Source: CAD feature listing. Evaluate the final solid. Frame: model axes, mm. Face numbers are marked on the shaded views. A direction names the side the tool comes from. Round coordinates to 2 decimals unless told otherwise and drop trailing zeros. Write each loop counter-clockwise with the first axis right and the second up, starting at its lowest first coordinate (ties: lowest second). Pieces come first, ordered by that corner, then holes. Notation, with made-up numbers: (-1, 8) -> (38, 8) arc R21 ccw to (38, 16) -> close; hole circle Ø2 at (40.25, 54.5). An arc over 180 degrees is marked (long way). Put each result on its own line as item: value.
Autodesk Inventor part; units mm, degrees
ref_plane "YZ Plane" through (0, 0, 0) normal (1, 0, 0) x (0, 1, 0)
ref_plane "XZ Plane" through (0, 0, 0) normal (0, 1, 0) x (-1, 0, 0)
ref_plane "XY Plane" through (0, 0, 0) normal (0, 0, 1) x (1, 0, 0)
sketch "Sketch1" plane through (0, 0, 0) normal (0, 1, 0) x (-1, 0, 0)
  line L0 (0, 0) -> (27, 0) construction
  line L1 (27, 0) -> (27, -25) construction
  line L2 (27, -25) -> (0, -25) construction
  line L3 (0, -25) -> (0, 0) construction
  line L4 (31, 2) -> (-4, 2)
  line L5 (-4, -27) -> (31, -27)
  line L6 (29, -22) -> (29, -3)
  line L7 (28, -4) -> (23.5, -4)
  line L8 (23.5, -4) -> (23.5, -21)
  line L9 (23.5, -21) -> (28, -21)
  line L10 (28, -21) -> (28, -4)
  arc A0 (31, -3) -> (31, 2) centre (31, -0.5) ccw
  arc A1 (31, -27) -> (31, -22) centre (31, -24.5) ccw
  arc A2 (-4, 2) -> (-4, -3) centre (-4, -0.5) ccw
  arc A3 (-4, -22) -> (-4, -27) centre (-4, -24.5) ccw
  line L11 (31, -3) -> (29, -3)
  line L12 (31, -22) -> (29, -22)
  line L13 (-4, -3) -> (-2, -3)
  line L14 (-4, -22) -> (-2, -22)
  line L15 (-2, -3) -> (-2, -22)
  circle A4 centre (31, -0.5) radius 1.35
  circle A5 centre (31, -24.5) radius 1.35
  circle A6 centre (-4, -0.5) radius 1.35
  circle A7 centre (-4, -24.5) radius 1.35
  point P0 (29, 2)
  point P1 (-2, -27)
  point P2 (-2, 2)
  point P3 (29, -27)
  dimension "d0" = 27
  dimension "d1" = 25
  dimension "d12" = 2
  dimension "d13" = 2
  dimension "d14" = 2
  dimension "d18" = 1
  dimension "d19" = 3.5
  dimension "d20" = 6
  dimension "d21" = 6
  dimension "d22" = 5
  dimension "d23" = 2.5
  dimension "d24" = 2
  dimension "d25" = 2.5
  dimension "d26" = 2
  dimension "d27" = 5
  dimension "d28" = 5
  dimension "d29" = 5
  dimension "d32" = 2.5
  dimension "d33" = 2.5
  dimension "d34" = 2.7
  dimension "d35" = 2.7
  dimension "d36" = 2.7
  dimension "d37" = 2.7
extrude "Extrusion1" add sketch "Sketch1" against normal blind 1
sketch "Sketch2" plane through (0, 0, 0) normal (0, 1, 0) x (1, 0, 0)
  line L0 (-31, -2) -> (4, -2)
  arc A0 (4, -2) -> (4, 3) centre (4, 0.5) ccw
  line L1 (4, 3) -> (2, 3)
  line L2 (2, 3) -> (2, 22)
  line L3 (2, 22) -> (4, 22)
  arc A1 (4, 22) -> (4, 27) centre (4, 24.5) ccw
  line L4 (4, 27) -> (-31, 27)
  arc A2 (-31, 27) -> (-31, 22) centre (-31, 24.5) ccw
  line L5 (-31, 22) -> (-29, 22)
  line L6 (-29, 22) -> (-29, 3)
  line L7 (-29, 3) -> (-31, 3)
  arc A3 (-31, 3) -> (-31, -2) centre (-31, 0.5) ccw
  circle A4 centre (4, 24.5) radius 1.35
  circle A5 centre (4, 0.5) radius 1.35
  circle A6 centre (-31, 24.5) radius 1.35
  circle A7 centre (-31, 0.5) radius 1.35
  line L8 (-28, 4) -> (-28, 21)
  line L9 (-28, 21) -> (-23.5, 21)
  line L10 (-23.5, 21) -> (-23.5, 4)
  line L11 (-23.5, 4) -> (-28, 4)
  line L12 (-28, 26) -> (1, 26)
  line L13 (1, 26) -> (1, -1)
  line L14 (1, -1) -> (-28, -1)
  line L15 (-28, -1) -> (-28, 26)
  point P0 (0, 0)
  dimension "d38" = 1
  dimension "d39" = 1
  dimension "d40" = 1
  dimension "d41" = 1
extrude "Extrusion2" add sketch "Sketch2" along normal blind 5
fillet "Fillet1" radius 2 4 edges at (2, 2, -3) (2, 2, -22) (-29, 2, -22) (-29, 2, -3)
sketch "Sketch4" plane through (0, 5, 0) normal (0, 1, 0) x (1, 0, 0)
  line L0 (-36.8851, 35.5263) -> (12.4576, 35.5263)
  line L1 (12.4576, 35.5263) -> (12.4576, 26.5)
  line L2 (12.4576, 26.5) -> (-36.8851, 26.5)
  line L3 (-36.8851, 26.5) -> (-36.8851, 35.5263)
  line L4 (4, 27) -> (-31, 27)
  point P0 (0, 0)
  dimension "d47" = 0.5
extrude "Extrusion3" cut sketch "Sketch4" against normal blind 10
sketch "Sketch5" plane through (0, 0, 0) normal (0, 1, 0) x (1, 0, 0)
  line L0 (1, -1) -> (-28, -1)
  line L1 (-28, -1) -> (1, -1)
  line L2 (1, -1) -> (1, 0.6)
  line L3 (1, 0.6) -> (-28, 0.6)
  line L4 (-28, 0.6) -> (-28, -1)
  line L5 (1, 26) -> (1, -1)
  line L6 (1, 26) -> (-28, 26)
  line L7 (1, -1) -> (-0.8, -1)
  line L8 (-0.8, -1) -> (-0.8, 26)
  line L9 (-0.8, 26) -> (1, 26)
  line L10 (1, 26) -> (1, -1)
  point P0 (0, 0)
  point P1 (-0.8, 0.6)
  dimension "d50" = 1.6
  dimension "d57" = 1.8
extrude "Extrusion4" add sketch "Sketch5" along normal up to surface (5 mm away)
sketch "Sketch6" plane through (0, -1, 0) normal (0, -1, 0) x (1, 0, 0)
  line L0 (-23.5, -4) -> (-28, -4)
  line L1 (-28, -0.6) -> (-28, -26)
  line L2 (-23.5, -4) -> (-28, -4)
  line L3 (-28, -4) -> (-28, -8)
  line L4 (-28, -8) -> (-23.5, -8)
  line L5 (-23.5, -8) -> (-23.5, -4)
  line L6 (-28, -21) -> (-23.5, -21)
  line L7 (-23.5, -4) -> (-25.6, -4)
  line L8 (-25.6, -4) -> (-25.6, -21)
  line L9 (-25.6, -21) -> (-23.5, -21)
  line L10 (-23.5, -21) -> (-23.5, -4)
  point P0 (0, 0)
  point P1 (-25.6, -8)
  dimension "d53" = 4
  dimension "d54" = 2.4
extrude "Extrusion5" add sketch "Sketch6" against normal up to surface (1 mm away) contours L5 L4 L8 L0 | L8 L4 L1 L0 | L10 L6 L8 L4
sketch "Sketch7" plane through (0, 0, 0) normal (0, 1, 0) x (1, 0, 0)
  line L0 (-28, 0.6) -> (-0.8, 0.6)
  line L1 (-0.8, 0.6) -> (-5.1, 0.6)
  line L2 (-5.1, 0.6) -> (-5.1, 4.9)
  line L3 (-5.1, 4.9) -> (-0.8, 4.9)
  line L4 (-0.8, 4.9) -> (-0.8, 0.6)
  line L5 (-28, 0.6) -> (-23.7, 0.6)
  line L6 (-23.7, 0.6) -> (-23.7, 4.9)
  line L7 (-23.7, 4.9) -> (-28, 4.9)
  line L8 (-28, 4.9) -> (-28, 0.6)
  line L9 (-28, 26) -> (-0.8, 26)
  line L10 (-28, 26) -> (-23.7, 26)
  line L11 (-23.7, 26) -> (-23.7, 21.7)
  line L12 (-23.7, 21.7) -> (-28, 21.7)
  line L13 (-28, 21.7) -> (-28, 26)
  line L14 (-0.8, 26) -> (-5.1, 26)
  line L15 (-5.1, 26) -> (-5.1, 21.7)
  line L16 (-5.1, 21.7) -> (-0.8, 21.7)
  line L17 (-0.8, 21.7) -> (-0.8, 26)
  point P0 (0, 0)
  point P1 (-0.8, 26)
  dimension "d58" = 4.3
  dimension "d59" = 4.3
  dimension "d60" = 4.3
  dimension "d61" = 4.3
  dimension "d62" = 4.3
  dimension "d63" = 4.3
extrude "Extrusion6" add sketch "Sketch7" along normal blind 1.86
fillet "Fillet2" radius 3 4 edges at (-23.7, 0.93, -21.7) (-23.7, 0.93, -4.9) (-5.1, 0.93, -21.7) (-5.1, 0.93, -4.9)
sketch "Sketch8" plane through (0, 0, 0) normal (0, 1, 0) x (1, 0, 0)
  line L0 (-28, 21.7) -> (-28, 26)
  line L1 (-28, 21.7) -> (-24.5334, 21.7)
  line L2 (-24.5334, 21.7) -> (-24.5334, 4.9)
  line L3 (-24.5334, 4.9) -> (-28, 4.9)
  line L4 (-28, 4.9) -> (-28, 21.7)
  point P0 (0, 0)
extrude "Extrusion7" cut sketch "Sketch8" against normal blind 10
equation "\"d13\" = d12"
equation "\"d14\" = d12"
equation "\"d15\" = d12"
properties part number "OledModBase"
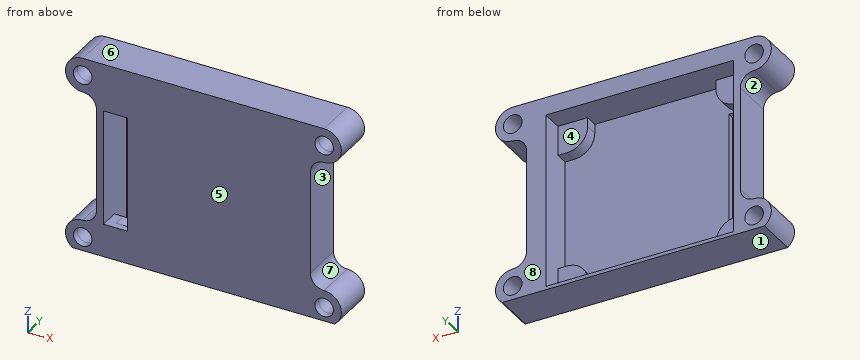
Q1. Pin query (flat end, axial travel): pin 1 (3 mm diameter, centred on y = 3, z = -16.5, fed in from +X); pin 2 (1 mm diameter, centred on y = 1, z = -9, fed in from -X); pin 3 (3.5 mm diameter, centred on x = -3.5, z = -2.5, fed in from +Y). Return the tip coordinate at first contact, or that it passes through.
Ans:
pin 1: stops at x = 2
pin 2: stops at x = -29
pin 3: stops at y = 1.86
Q2. Cut plane C-C on x = -23. Output: boundary loops of the cut face in (y, z), and give its area (3 significant figures).
Ans:
outline: (-1, -26.5) -> (5, -26.5) -> (5, -26) -> (0, -26) -> (0, -0.6) -> (5, -0.6) -> (5, 2) -> (-1, 2) -> close
area: 44.0 mm^2
Q3. Draft query along Z for the marked faces 6, 7 and 8. Return one class per face: +Z half, -Z half, draft (parallel to the pull), parting line (faces both ways), or undercut.
Ans:
face 6: +Z half
face 7: undercut
face 8: draft
Q4. Cut plane A-A on z = -15.75. Output: boundary loops of the cut face in (x, y).
Ans:
outline: (-29, -1) -> (-28, -1) -> (-28, 5) -> (-29, 5) -> close; (-24.53, -1) -> (2, -1) -> (2, 5) -> (-0.8, 5) -> (-0.8, 0) -> (-24.53, 0) -> close
Q5. Cut plane B-B on y = 4.55. Give the number of separate pieces and of enclosed holes in the cut face, and give its area (3 significant figures).
Ans:
separate pieces: 1
enclosed holes: 5
area: 249 mm^2
Q6. Material intervals for line 1 (X direction, y = 3.05, z = -0.5); line 2 (Z direction, x = 4, y = 1.2); line 3 (X direction, y = 3.6, z = -24.5), sorted ascending. Write a range as [from, to].
Ans:
line 1: x = [-33.5, -32.35], [-29.65, 2.65], [5.35, 6.5]
line 2: z = [-26.5, -25.85], [-23.15, -22], [-3, -1.85], [0.85, 2]
line 3: x = [-33.5, -32.35], [-29.65, -28], [-0.8, 2.65], [5.35, 6.5]
Q7. Reachability of the marked faces 1, 2, 3, 4 and 5 from +Z, -Z, +X, -X, +Y, -Y: full face, straight path, thin tool, end or side. Return the list, or none.
Ans:
face 1: -Z, +X, -X, +Y, -Y
face 2: -X, +Y, -Y
face 3: +X, +Y, -Y
face 4: +Y
face 5: +Z, -Z, +X, -X, -Y
Q8. Cut plane D-D on z = -24. Output: boundary loops of the cut face in (x, y).
Ans:
outline: (-33.45, -1) -> (-32.25, -1) -> (-32.25, 5) -> (-33.45, 5) -> close; (-29.75, -1) -> (2.75, -1) -> (2.75, 5) -> (-0.8, 5) -> (-0.8, 1.86) -> (-5.02, 1.86) -> (-5.02, 0) -> (-23.78, 0) -> (-23.78, 1.86) -> (-28, 1.86) -> (-28, 5) -> (-29.75, 5) -> close; (5.25, -1) -> (6.45, -1) -> (6.45, 5) -> (5.25, 5) -> close
